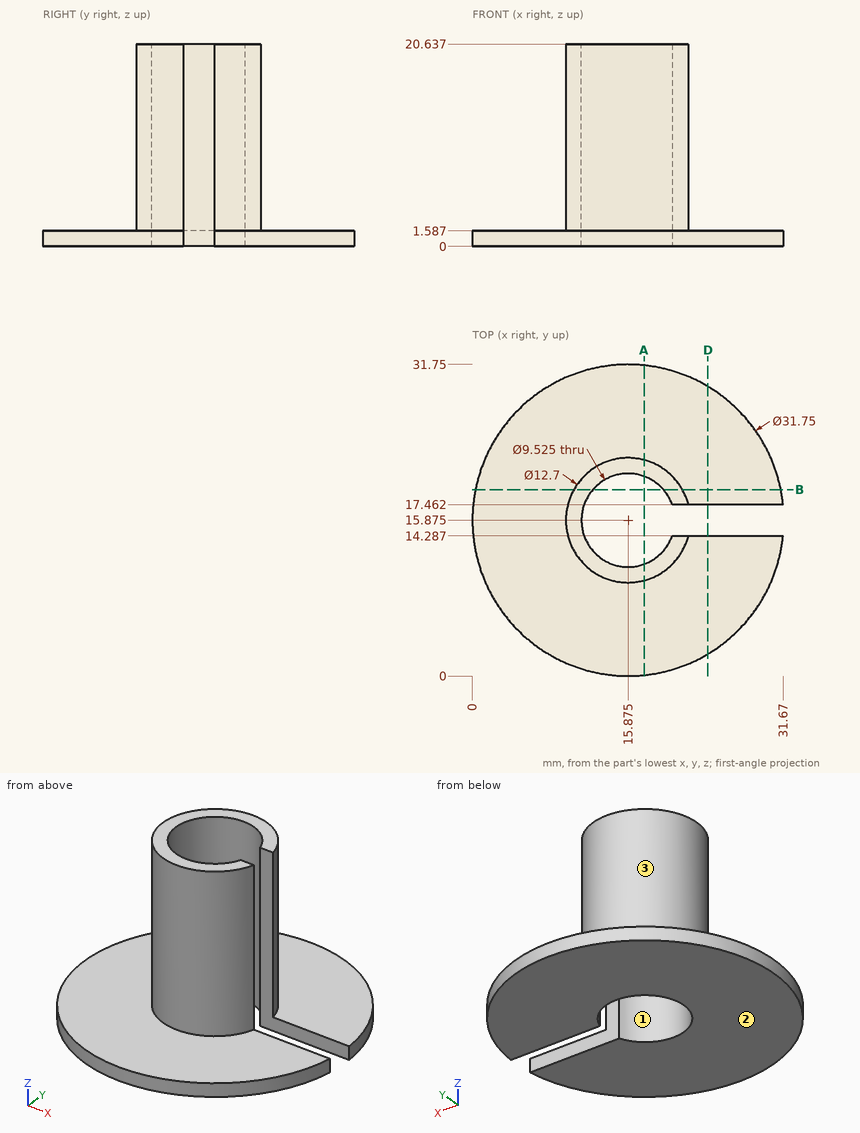
For this review, use the dimensioned drawing (mm, ordinates from the lowest corner) and the shaded views. Coordinates: 2 decimals unless noted, no trailing zeros. Loops run counter-clockwise (first coordinate to the right, second up) from the corner with the lowest first, then second, coordinate; pieces in that order, holes last. Notation, with made-up numbers: (-36, 60.25) -> (-13, 60.25) arc R19 cw to (-13, 70.25) -> close; hole circle Ø9 at (-9, 36). An arc over 180 degrees is marked (long way). Return JSON: item names as keys, results as strings. Group by question number.
(1) To check wall thickness, follow L1, parallel to Z at x = 6, y = 14; L2, parallel to X at y = 12.5, z = 10.75 (1 decimal); L3, parallel to Y at x = 19, z = 6.25 (1 decimal). State the ranges of each line that lie inside material, in increasing order.
(2) Mouldability with a two-part tool opening along X and no side actions: class the marked faces 1, 2 and 3 as pulls with the +X half, pulls with the -X half, needs draft (parallel to the pull), parting line crosses it, or undercut.
(3) For pin 1 Ø10 at (y, z) = (11, 14) entering from -X (1 decimal); pin 2 Ø9 at (x, z) = (24.5, 14) entering from +Y; pin 3 Ø5 at (x, z) = (21, 8.5) entering from -Y, all flat-tipped, find the tip position at first contact; note any pin that passes through.
(4) Consider section A-A, the plane x = 17.5. Give the boundary of the cut face in (y, z).
(5) Consider section D-D, the plane x = 24. Give the boundary of the cut face in (y, z).
(6) Consider section B-B, the plane y = 19. Give the boundary of the cut face in (x, z).
Results below:
{
 "1": {"L1": "z = 0 to 1.59", "L2": "x = 10.5 to 12.5, 19.2 to 21.3", "L3": "y = 10.3 to 12.3, 19.5 to 21.4"},
 "2": {"face 1": "undercut", "face 2": "needs draft", "face 3": "parting line crosses it"},
 "3": {"pin 1": "stops at x = 9.5", "pin 2": "stops at y = 20.7", "pin 3": "stops at y = 10.09"},
 "4": {"outline": "(0.08, 0) -> (11.4, 0) -> (11.4, 20.64) -> (9.74, 20.64) -> (9.74, 1.59) -> (0.08, 1.59) -> close; (20.35, 0) -> (31.67, 0) -> (31.67, 1.59) -> (22.01, 1.59) -> (22.01, 20.64) -> (20.35, 20.64) -> close"},
 "5": {"outline": "(2.24, 0) -> (14.29, 0) -> (14.29, 1.59) -> (2.24, 1.59) -> close; (17.46, 0) -> (29.51, 0) -> (29.51, 1.59) -> (17.46, 1.59) -> close"},
 "6": {"outline": "(0.31, 0) -> (12.28, 0) -> (12.28, 20.64) -> (10.35, 20.64) -> (10.35, 1.59) -> (0.31, 1.59) -> close; (19.47, 0) -> (31.44, 0) -> (31.44, 1.59) -> (21.4, 1.59) -> (21.4, 20.64) -> (19.47, 20.64) -> close"}
}
